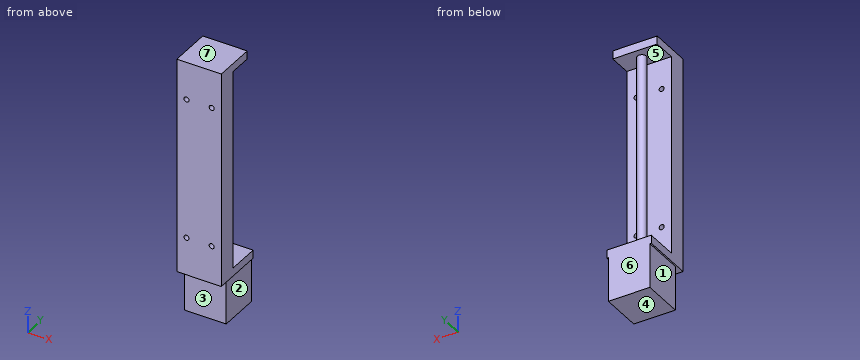
Autodesk Inventor part; units mm, degrees
ref_plane "YZ Plane" through (0, 0, 0) normal (1, 0, 0) x (0, 1, 0)
ref_plane "XZ Plane" through (0, 0, 0) normal (0, 1, 0) x (-1, 0, 0)
ref_plane "XY Plane" through (0, 0, 0) normal (0, 0, 1) x (1, 0, 0)
sketch "Sketch1" plane through (0, 0, 0) normal (0, 1, 0) x (-1, 0, 0)
  line L0 (0, 0) -> (30, 0)
  line L1 (30, 0) -> (30, -146)
  line L2 (30, -146) -> (0, -146)
  line L3 (0, -146) -> (0, 0)
  dimension "d0" = 30
  dimension "d1" = 146
extrude "Extrusion1" add sketch "Sketch1" along normal blind 13
sketch "Sketch2" plane through (0, 13, 0) normal (0, 1, 0) x (1, 0, 0)
  line L0 (-30, 146) -> (-30, 0)
  line L1 (0, 0) -> (0, 146)
  line L2 (-30, 0) -> (0, 0)
  line L3 (0, 0) -> (0, 5.5)
  line L4 (0, 5.5) -> (-30, 5.5)
  line L5 (-30, 5.5) -> (-30, 0)
  line L6 (0, 146) -> (-30, 146)
  line L7 (-30, 146) -> (-30, 140.5)
  line L8 (-30, 140.5) -> (0, 140.5)
  line L9 (0, 140.5) -> (0, 146)
  line L10 (-30, 146) -> (0, 146)
  line L11 (0, 146) -> (0, 140.5)
  line L12 (0, 140.5) -> (-30, 140.5)
  line L13 (-30, 140.5) -> (-30, 146)
  dimension "d4" = 5.5
  dimension "d5" = 5.5
extrude "Extrusion2" add sketch "Sketch2" along normal blind 15.5 contours L4 L1 L2 L0
sketch "Sketch4" plane through (0, 13, 0) normal (0, 1, 0) x (1, 0, 0)
  line L0 (0, 0) -> (0, 146)
  line L1 (-30, 146) -> (-30, 0)
  line L2 (0, 146) -> (-30, 146)
  line L3 (-30, 146) -> (-30, 140.5)
  line L4 (-30, 140.5) -> (0, 140.5)
  line L5 (0, 140.5) -> (0, 146)
  point P0 (0, 140.5)
  dimension "d8" = 5.5
extrude "Extrusion3" add sketch "Sketch4" along normal blind 22
sketch "Sketch6" plane through (0, 0, -146) normal (0, 0, -1) x (-1, 0, 0)
  line L0 (30, 35) -> (0, 35) construction
  line L1 (30, 0) -> (30, 28.5)
  line L2 (0, 35) -> (30, 35) construction
  line L3 (30, 35) -> (30, 7) construction
  line L4 (30, 7) -> (0, 7) construction
  line L5 (0, 7) -> (0, 35) construction
  line L6 (0, 7) -> (30, 35) construction
  line L7 (0, 35) -> (30, 7) construction
  circle A0 centre (15, 21) radius 3
  point P0 (0, 0)
  dimension "d11" = 28
  dimension "d12" = 6
extrude "Extrusion4" add sketch "Sketch6" against normal up to surface (140.5 mm away)
sketch "Sketch7" plane through (0, 0, -146) normal (0, 0, -1) x (-1, 0, 0)
  line L0 (30, 0) -> (30, 28.5)
  line L1 (30, 35) -> (0, 35)
  line L2 (1, 35) -> (29, 35)
  line L3 (29, 35) -> (29, 7)
  line L4 (29, 7) -> (1, 7)
  line L5 (1, 7) -> (1, 35)
  point P0 (0, 0)
  point P1 (15, 35)
  dimension "d15" = 28
extrude "Extrusion5" add sketch "Sketch7" along normal blind 30
sketch "Sketch8" plane through (0, 0, 0) normal (0, -1, 0) x (1, 0, 0)
  circle A0 centre (-6.5, -120.5) radius 1.7
  circle A1 centre (-23.5, -120.5) radius 1.7
  circle A2 centre (-6.5, -25.5) radius 1.7
  circle A3 centre (-23.5, -25.5) radius 1.7
  line L0 (0, 0) -> (0, -146)
  line L1 (-30, 0) -> (0, 0)
  line L2 (-30, -146) -> (-30, 0)
  line L3 (0, -146) -> (-30, -146)
  dimension "d18" = 3.4
  dimension "d19" = 95
  dimension "d20" = 6.5
  dimension "d21" = 25.5
  dimension "d22" = 6.5
  dimension "d25" = 17
  dimension "d26" = 25.5
extrude "Extrusion6" cut sketch "Sketch8" against normal blind 30 contours A0 | A1 | A2 | A3
equation "\"d5\" = d4"
equation "\"d22\" = d20"
properties part number "AE_100MM_STAGE"
Geometry: final body of the model. Coordinates: model frame, mm. Face numbers are marked on the shaded views. A direction names the side the tool comes from. Round coordinates to 2 decimals unless told otherwise and drop trailing zeros. Write each loop counter-clockwise with the first axis right and the second up, starting at its lowest first coordinate (ties: lowest second). Pieces come first, ordered by that corner, then holes.
Item 1: Mould query, pull axis Z, two halves, no side actions, for the marked faces 4, 5, 6 and 7. Classes: +Z half, -Z half, draft (parallel to the pull), parting line (faces both ways), or undercut.
Item 2: Set-up query: the marked faces 1, 2 and 3. Return all of +Z, -Z, +X, -X, +Y, -Y with unobstructed straight access to the full face (end or side cutting, diameter ignored); none if empty.
Item 3: Material intervals for L1, parallel to Z at x = -23.5, y = 2.75; L2, parallel to Z at x = -23.5, y = 10; L3, parallel to X at y = 7.5, z = -120.5, sorted ascending.
Item 4: Pin query (flat end, axial travel): P1, Ø2, axis at x = -10, y = 31, coming from the +Z side; P2, Ø14, axis at x = -15, z = -165.5, coming from the -Y side; P3, Ø6, axis at x = -12, z = -3, coming from the +Y side; P4, Ø2, axis at x = -23.5, z = -25.5, coming from the +Y side. Return the tip coordinate at first contact, or that it passes through.
Item 5: Section query B-B (y = 2.5). Return loops of the section in (x, z).
Item 6: Section query A-A (x = -23.5). Return loops of the section in (y, z), plus the area to 3 significant figures.
Item 7: Section query D-D (z = -94). Return loops of the section in (x, y), plus the area to 3 significant figures.
Item 8: Section query C-C (z = -120.5). Return loops of the section in (x, y).
Completed:
1. face 4: -Z half
1. face 5: undercut
1. face 6: draft
1. face 7: +Z half
2. face 1: -Z, -X, +Y, -Y
2. face 2: -Z, +X, +Y, -Y
2. face 3: -Z, +X, -X, -Y
3. L1: z = -146 to -122.2, -118.8 to -27.2, -23.8 to 0
3. L2: z = -176 to -122.2, -118.8 to -27.2, -23.8 to 0
3. L3: x = -30 to -25.2, -21.8 to -8.2, -4.8 to 0
4. P1: stops at z = -140.5
4. P2: stops at y = 7
4. P3: stops at y = 28.5
4. P4: passes through
5. outline: (-30, -146) - (0, -146) - (0, 0) - (-30, 0) - close; hole circle Ø3.4 at (-23.5, -120.5); hole circle Ø3.4 at (-23.5, -25.5); hole circle Ø3.4 at (-6.5, -120.5); hole circle Ø3.4 at (-6.5, -25.5)
6. outline: (0, -146) - (7, -146) - (7, -176) - (35, -176) - (35, -140.5) - (13, -140.5) - (13, -122.2) - (0, -122.2) - close; (0, -118.8) - (13, -118.8) - (13, -27.2) - (0, -27.2) - close; (0, -23.8) - (13, -23.8) - (13, -5.5) - (28.5, -5.5) - (28.5, 0) - (0, 0) - close
6. area: 2,860 mm2
7. outline: (-30, 0) - (0, 0) - (0, 13) - (-30, 13) - close; circle Ø6 at (-15, 21)
7. area: 418 mm2
8. outline: (-30, 0) - (-25.2, 0) - (-25.2, 13) - (-30, 13) - close; (-21.8, 0) - (-8.2, 0) - (-8.2, 13) - (-21.8, 13) - close; circle Ø6 at (-15, 21); (-4.8, 0) - (0, 0) - (0, 13) - (-4.8, 13) - close
